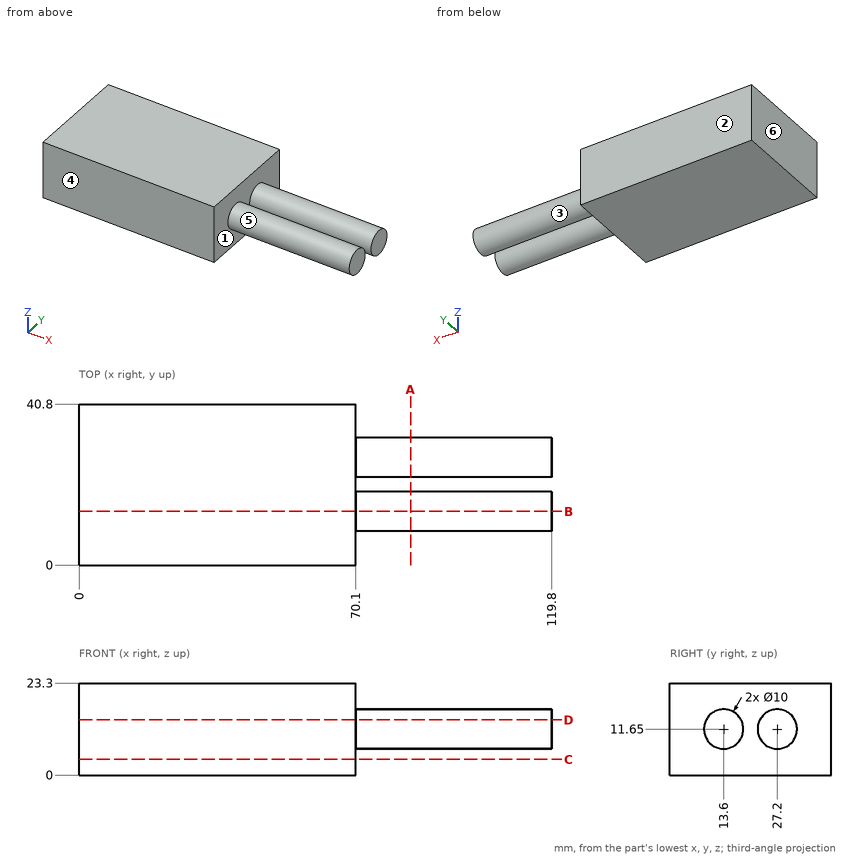
Can you work these out from the drawing? Everything is in mm from the part's minimum corner. A direction names the side the tool comes from. Round coordinates to 2 decimals unless told otherwise and drop trailing zeros. Loops run counter-clockwise (first coordinate to the right, second up) from the corner with the lowest first, then second, coordinate; pieces in that order, holes last. Notation, with made-up numbers: (38, 64.25) - (75, 64.25) arc R16 ccw to (75, 92.25) - close; hole circle Ø9 at (64, 13.25). An arc over 180 degrees is marked (long way). Answer in a Markdown table with one row per item. Add a question column.
Q1. I want a section at B-B on y = 13.6. List the corners of the cut face in (x, z) for me.
Q2. I need wall thicknesses on L1, parallel to X at y = 4.5, z = 3; L2, parallel to Y at x = 77.5, z = 7.5; L3, parallel to Y at x = 96, z = 8.5. Which ranges of each line are inside material? Lowest first, please.
Q3. I want a section at D-D on z = 14. List the corners of the cut face in (x, y) for me.
Q4. We'd pull the mould along Y, two halves only. Please class the marked faces 3, 4, 5 and 6: pulls with the +Y half, pulls with the -Y half, needs draft (parallel to the pull), parting line crosses it, or undercut.
Q5. I want a section at C-C on z = 4. List the corners of the cut face in (x, y) for me, and give its area (3 significant figures).
Q6. Which directions (+Z, -Z, +X, -X, +Y, -Y) give clear straight access to the entire face, cutting with the end or side of a thin tool? Please do the marked faces 1 and 2.
Q7. For pin 1 Ø2 at (y, z) = (16, 3) entering from +X; pin 2 Ø1 at (x, y) = (97.5, 11) entering from +Z; pin 3 Ø5 at (x, y) = (87.5, 27.5) entering from -Z, each with a flat end and sliding along its axis, tell me the tip position at first contact or that it passes through.
Q8. I want a section at A-A on x = 84. List the corners of the cut face in (y, z) for me, and give its area (3 significant figures).
A:
| question | item | result |
|---|---|---|
| 1 | outline | (0, 0) - (70.1, 0) - (70.1, 6.65) - (119.8, 6.65) - (119.8, 16.65) - (70.1, 16.65) - (70.1, 23.3) - (0, 23.3) - close |
| 2 | L1 | 0 to 70.1 |
| 2 | L2 | 10.81 to 16.39, 24.41 to 29.99 |
| 2 | L3 | 9.72 to 17.48, 23.32 to 31.08 |
| 3 | outline | (0, 0) - (70.1, 0) - (70.1, 9.19) - (119.8, 9.19) - (119.8, 18.01) - (70.1, 18.01) - (70.1, 22.79) - (119.8, 22.79) - (119.8, 31.61) - (70.1, 31.61) - (70.1, 40.8) - (0, 40.8) - close |
| 4 | face 3 | undercut |
| 4 | face 4 | pulls with the -Y half |
| 4 | face 5 | undercut |
| 4 | face 6 | needs draft |
| 5 | outline | (0, 0) - (70.1, 0) - (70.1, 40.8) - (0, 40.8) - close |
| 5 | area | 2,860 mm^2 |
| 6 | face 1 | +X |
| 6 | face 2 | +Z, -Z, +X, -X, +Y |
| 7 | pin 1 | x = 70.1 |
| 7 | pin 2 | z = 16.19 |
| 7 | pin 3 | z = 6.65 |
| 8 | outline | circle Ø10 at (13.6, 11.65); circle Ø10 at (27.2, 11.65) |
| 8 | area | 157 mm^2 |
